from build123d import *

# Parameters (mm, degrees)
SKETCH1_W           = 20
SKETCH1_H           = 30
BOSS_EXTRUDE1_DEPTH = 20
SKETCH2_W           = 20
SKETCH2_H           = 8
BOSS_EXTRUDE2_DEPTH = 10
SKETCH3_W           = 20
SKETCH3_H           = 8
BOSS_EXTRUDE3_DEPTH = 10
SKETCH4_R           = 2
CUT_EXTRUDE1_DEPTH  = 10
SKETCH5_R           = 6
CUT_EXTRUDE3_DEPTH  = 10
SKETCH6_R           = 2
CUT_EXTRUDE4_DEPTH  = 10
SKETCH7_W           = 15
SKETCH7_H           = 5
CUT_EXTRUDE5_DEPTH  = 10


with BuildPart() as part:
    # Sketch1 → Boss-Extrude1 (new body)
    with BuildSketch(Plane.XY):
        Rectangle(SKETCH1_W, SKETCH1_H)
    extrude(amount=BOSS_EXTRUDE1_DEPTH)

    # Sketch2 → Boss-Extrude2 (add)
    with BuildSketch(Plane.ZY.offset(10)):
        with Locations((10, 11)):
            Rectangle(SKETCH2_W, SKETCH2_H)
    extrude(amount=BOSS_EXTRUDE2_DEPTH)

    # Sketch3 → Boss-Extrude3 (add)
    with BuildSketch(Plane(origin=(10, 0, 0), x_dir=(0, 0, -1), z_dir=(1, 0, 0))):
        with Locations((-10, 11)):
            Rectangle(SKETCH3_W, SKETCH3_H)
    extrude(amount=BOSS_EXTRUDE3_DEPTH)

    # Sketch4 → Cut-Extrude1 (cut)
    with BuildSketch(Plane(origin=(0, 15, 0), x_dir=(1, 0, 0), z_dir=(0, 1, 0))):
        with Locations(Location((-15, -7.5, 0), (0, 0, 270))):
            Circle(SKETCH4_R)
        with Locations(Location((15, -7.5, 0), (0, 0, 270))):
            Circle(SKETCH4_R)
    extrude(amount=-CUT_EXTRUDE1_DEPTH, mode=Mode.SUBTRACT)

    # Sketch5 → Cut-Extrude3 (cut)
    with BuildSketch(Plane(origin=(0, 0, 0), x_dir=(-1, 0, 0), z_dir=(0, 0, -1))):
        with Locations((0, 1.296765848)):
            Circle(SKETCH5_R)
    extrude(amount=-CUT_EXTRUDE3_DEPTH, mode=Mode.SUBTRACT)

    # Sketch6 → Cut-Extrude4 (cut)
    with BuildSketch(Plane(origin=(0, 0, 10), x_dir=(-1, 0, 0), z_dir=(0, 0, -1))):
        Circle(SKETCH6_R)
    extrude(amount=-CUT_EXTRUDE4_DEPTH, mode=Mode.SUBTRACT)

    # Sketch7 → Cut-Extrude5 (cut)
    with BuildSketch(Plane(origin=(20, 0, 0), x_dir=(0, 0, -1), z_dir=(1, 0, 0))):
        with Locations((-10.063514781, 11.051610094)):
            Rectangle(SKETCH7_W, SKETCH7_H)
    extrude(amount=-CUT_EXTRUDE5_DEPTH, mode=Mode.SUBTRACT)


solid = part.part
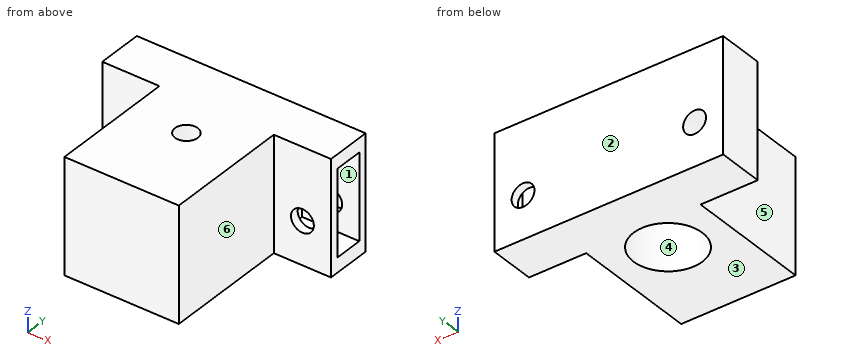
Geometry: final body of the model. Coordinates: model frame, mm. Face numbers are marked on the shaded views. A direction names the side the tool comes from. Give positions to 0.01 mm unless a question says otherwise; leave off trailing zeros. Loops run counter-clockwise (first coordinate to the right, second up) from the corner with the lowest first, then second, coordinate; pieces in that order, holes last. Notation, with made-up numbers: (69.5, -12) - (86.5, -12) arc R33 cw to (86.5, 24) - close; hole circle Ø1 at (59, -0.75). An arc over 180 degrees is marked (long way). One line per question, with ' | ' between items. Start each with the question number.
(1) Section query D-D on x = -15. Return loops of the section in (y, z), then the cut area to 3 significant figures.
(2) Pull-direction query (Y, two-part tool) for the marked faces 1, 2 and 3; classes: released by +Y, released by -Y, zero draft, split by the parting line, or undercut.
(3) Section query B-B on z = 11. Return loops of the section in (x, y).
(4) Section query C-C on z = 7.5. Return loops of the section in (x, y).
(5) Reachability of the marked faces 4, 5 and 6 from +Z, -Z, +X, -X, +Y, -Y: full face, straight path, thin tool, end or side. Return the list, or none.
(6) Section query A-A on x = 15. Return loops of the section in (y, z), then the cut area to 3 significant figures.
(7) Ray query, line 1 (X direction, y = 14.4, z = 7.5); line 2 (Y direction, x = 17, z = 10); line 3 (Z direction, x = 15, y = 11.25). Return the intervals inside material, ascending. Write a range as from..to.
(8) Contact query for flat-ended pins moving along their axis: pin 1 (4.5 mm diameter, centred on x = 15, z = 7.5, fed in from -Y); pin 2 (1 mm diameter, centred on y = 2, z = 14, fed in from -X); pin 3 (10 mm diameter, centred on y = -1, z = 13, fed in from +X). Output: stop coordinate, or through.
The answers:
1) outline: (7, 0) - (15, 0) - (15, 5.5) - (7, 5.5) - close; (7, 9.5) - (15, 9.5) - (15, 20) - (7, 20) - close | area: 128 mm2
2) face 1: undercut | face 2: released by +Y | face 3: zero draft
3) outline: (-20, 7) - (-10, 7) - (-10, -15) - (10, -15) - (10, 7) - (20, 7) - (20, 8.55) - (10, 8.55) - (10, 13.55) - (20, 13.55) - (20, 15) - (-20, 15) - close; hole circle Ø4 at (0, 0)
4) outline: (-20, 7) - (-17, 7) - (-17, 15) - (-20, 15) - close; (-13, 7) - (-10, 7) - (-10, -15) - (10, -15) - (10, 7) - (13, 7) - (13, 8.55) - (10, 8.55) - (10, 13.55) - (13, 13.55) - (13, 15) - (-13, 15) - close; (17, 7) - (20, 7) - (20, 8.55) - (17, 8.55) - close; (17, 13.55) - (20, 13.55) - (20, 15) - (17, 15) - close; hole circle Ø12 at (0, 1.3)
5) face 4: -Z | face 5: +Z, -Z, -X, -Y | face 6: +Z, -Z, +X, -Y
6) outline: (7, 0) - (15, 0) - (15, 5.5) - (13.55, 5.5) - (13.55, 2.56) - (8.55, 2.56) - (8.55, 5.5) - (7, 5.5) - close; (7, 9.5) - (8.55, 9.5) - (8.55, 17.56) - (13.55, 17.56) - (13.55, 9.5) - (15, 9.5) - (15, 20) - (7, 20) - close | area: 73.0 mm2
7) line 1: -20..-17, -13..13, 17..20 | line 2: 7..8.55, 13.55..15 | line 3: 0..2.56, 17.56..20
8) pin 1: y = 7 | pin 2: x = -10 | pin 3: x = 10
